The figure shows three views and two pictorial views of one solid part (mm, origin at its lowest corner). Answer the questions. Give positions to 0.01 mm unless a question says otherwise; leave off trailing zeros. Order: outer loops, then holes, each group sorted by start corner. A loop starts at its lowest first (then second) coordinate and runs counter-clockwise, first axis right, second up. Notation, with made-up numbers: (6, 51) - (48, 51) arc R15 ccw to (48, 68) - close; hole circle Ø4 at (47.25, -12.75). An arc over 180 degrees is marked (long way). Use a Markdown table: item, result. Add a question column.
1. A cutting plane is placed at A-A on y = 0.4. Determine the outline of the cut face in (x, z), and give its area (3 significant figures).
2. A cutting plane is placed at C-C on z = 9. Determine the outline of the cut face in (x, y), and give its area (3 significant figures).
3. A cutting plane is placed at B-B on x = 14.5. Determine the outline of the cut face in (y, z), and give its area (3 significant figures).
4. Consider L1, parallel to X at y = 0.75, z = 8; L2, parallel to Z at x = 1.25, y = 1.5; L3, parallel to X at y = 0.9, z = 0.5. Determine where each line is inside the solid, lowest interval first.
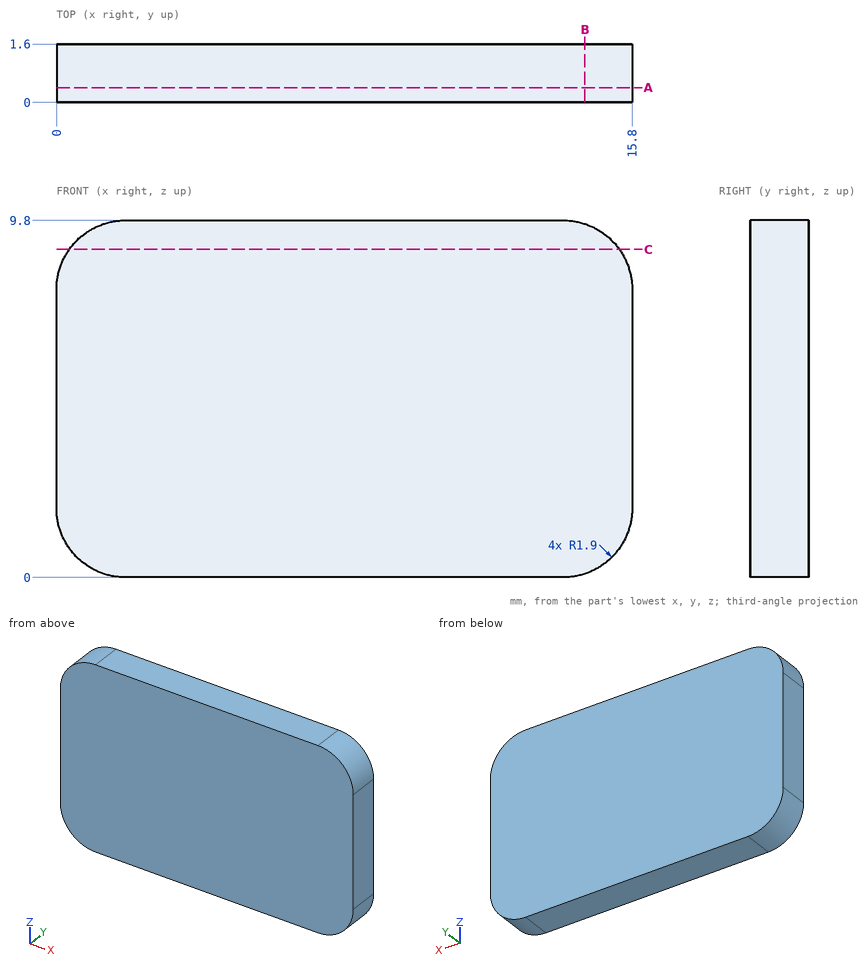
Output values:
| question | item | result |
|---|---|---|
| 1 | outline | (0, 1.9) arc R1.9 ccw to (1.9, 0) - (13.9, 0) arc R1.9 ccw to (15.8, 1.9) - (15.8, 7.9) arc R1.9 ccw to (13.9, 9.8) - (1.9, 9.8) arc R1.9 ccw to (0, 7.9) - close |
| 1 | area | 152 mm² |
| 2 | outline | (0.35, 0) - (15.45, 0) - (15.45, 1.6) - (0.35, 1.6) - close |
| 2 | area | 24.2 mm² |
| 3 | outline | (0, 0.1) - (1.6, 0.1) - (1.6, 9.7) - (0, 9.7) - close |
| 3 | area | 15.4 mm² |
| 4 | L1 | 0 to 15.8 |
| 4 | L2 | 0.11 to 9.69 |
| 4 | L3 | 0.62 to 15.18 |
